Verification items for the finished model (mm, model axes). A direction names the side the tool comes from. Give positions to 0.01 mm unless a question says otherwise; leave off trailing zeros. Write each loop counter-clockwise with the first axis right and the second up, starting at its lowest first coordinate (ties: lowest second). Pieces come first, ordered by that corner, then holes. Notation, with made-up numbers: (-31.5, 89.5) -> (17.5, 89.5) arc R23 ccw to (17.5, 115.5) -> close; hole circle Ø1 at (-20, 54.25). An arc over 180 degrees is marked (long way). Use CSV: the item, a comma, the result in double quotes. Start each with the question number.
```python
from build123d import *

# Parameters (mm, degrees)
F0_R     = 12.5
F1_DEPTH = 20
F2_DEPTH = 45.3


with BuildPart() as f1:
    # F0 (on Front) → F1 (new body)
    with BuildSketch(Plane.XZ):
        with BuildLine():
            ThreePointArc((2.5, 24.874686), (18.540496, 16.77051), (25, 0))
            ThreePointArc((25, 0), (18.540496, -16.77051), (2.5, -24.874686))
            Line((2.5, -24.874686), (101.5, -14.924812))
            ThreePointArc((101.5, -14.924812), (85, 0), (101.5, 14.924812))
            Line((101.5, 14.924812), (2.5, 24.874686))
        make_face()
        with BuildLine():
            ThreePointArc((2.5, -24.874686), (18.540496, -16.77051), (25, 0))
            ThreePointArc((25, 0), (18.540496, 16.77051), (2.5, 24.874686))
            ThreePointArc((2.5, 24.874686), (-25, 0), (2.5, -24.874686))
        make_face()
        with BuildLine():
            ThreePointArc((-11.456439, 5), (0, 12.5), (11.456439, 5))
            Line((11.456439, 5), (15, 5))
            Line((15, 5), (15, -5))
            Line((15, -5), (11.456439, -5))
            ThreePointArc((11.456439, -5), (0, -12.5), (-11.456439, -5))
            Line((-11.456439, -5), (-15, -5))
            Line((-15, -5), (-15, 5))
            Line((-15, 5), (-11.456439, 5))
        make_face(mode=Mode.SUBTRACT)
        with BuildLine():
            ThreePointArc((115, 0), (111.124298, 10.062306), (101.5, 14.924812))
            ThreePointArc((101.5, 14.924812), (85, 0), (101.5, -14.924812))
            ThreePointArc((101.5, -14.924812), (111.124298, -10.062306), (115, 0))
        make_face()
        with Locations((100, 0)):
            Circle(F0_R, mode=Mode.SUBTRACT)
        with BuildLine():
            ThreePointArc((-11.456439, -5), (-12.5, 0), (-11.456439, 5))
            Line((-11.456439, 5), (-15, 5))
            Line((-15, 5), (-15, -5))
            Line((-15, -5), (-11.456439, -5))
        make_face()
    extrude(amount=F1_DEPTH)

    # F0 (on Front) → F2 (join)
    with BuildSketch(Plane.XZ):
        with BuildLine():
            ThreePointArc((2.5, -24.874686), (18.540496, -16.77051), (25, 0))
            ThreePointArc((25, 0), (18.540496, 16.77051), (2.5, 24.874686))
            ThreePointArc((2.5, 24.874686), (-25, 0), (2.5, -24.874686))
        make_face()
        with BuildLine():
            ThreePointArc((-11.456439, 5), (0, 12.5), (11.456439, 5))
            Line((11.456439, 5), (15, 5))
            Line((15, 5), (15, -5))
            Line((15, -5), (11.456439, -5))
            ThreePointArc((11.456439, -5), (0, -12.5), (-11.456439, -5))
            Line((-11.456439, -5), (-15, -5))
            Line((-15, -5), (-15, 5))
            Line((-15, 5), (-11.456439, 5))
        make_face(mode=Mode.SUBTRACT)
        with BuildLine():
            ThreePointArc((-11.456439, -5), (-12.5, 0), (-11.456439, 5))
            Line((-11.456439, 5), (-15, 5))
            Line((-15, 5), (-15, -5))
            Line((-15, -5), (-11.456439, -5))
        make_face()
    extrude(amount=F2_DEPTH)


solid = f1.part
```
(1) Thickness scan on line 1 (X direction, y = -19.5, z = -6); line 2 (Y direction, x = 29, z = 20); line 3 (Z direction, x = 100, y = -13.75). Record the ranges inside material, lowest first. Write a range as from..to.
(2) Draft check along Z on faces 1 (the face through (51, -10, -20)), 2 (the face through (111.923, -9.86, 3.755)), 3 (the face through (15, -22, 0)), 4 (the face through (-11.5, -45.3, 5.9)). Enter one of: released by +Z, released by -Z, zero draft, split by the parting line, or undercut.
(3) Section check C-C on z = -18.5. Record the cut outline in (x, y), then the cut area to 3 significant figures.
(4) Section check A-A on x = 6. Record the cut outline in (y, z).
(5) Go/stop test with flat-tipped pins: pin 1 (1.8 mm diameter, centred on x = 12.5, y = -29, fed in from -Z); pin 2 (6 mm diameter, centred on y = -14.5, z = 6.5, fed in from +X); pin 3 (22.5 mm diameter, centred on x = 100, z = 0, fed in from +Y); pin 4 (25 mm diameter, centred on x = 80.5, z = 9.5, fed in from -Y). Record where each tip stops, or that it passes through.
(6) Section check B-B on y = -15.5. Record the cut outline in (x, z).
(7) Set-up check for faces 5 (the face through (13, -22, 5)), 6 (the face through (28, 0, 0)): record each of +Z, -Z, +X, -X, +Y, -Y from which the full face is reachable in a straight line by a thin tool's end or side.
(8) Section check D-D on x = 20.5. Record the cut outline in (y, z), then the cut area to 3 significant figures.
Data:
1,line 1,"x = -24.27..-10.97, 10.97..89.03, 110.97..113.75"
1,line 2,"y = -20..0"
1,line 3,"z = -15.08..-12.5, 12.5..15.08"
2,face 1,"released by -Z"
2,face 2,"undercut"
2,face 3,"undercut"
2,face 4,"zero draft"
3,outline,"(-16.82, -45.3) -> (16.82, -45.3) -> (16.82, -20) -> (65.93, -20) -> (65.93, 0) -> (-16.82, 0) -> close"
3,area,"2,510 mm2"
4,outline,"(-45.3, -24.27) -> (-20, -24.27) -> (-20, -24.52) -> (0, -24.52) -> (0, -10.97) -> (-45.3, -10.97) -> close; (-45.3, 10.97) -> (0, 10.97) -> (0, 24.52) -> (-20, 24.52) -> (-20, 24.27) -> (-45.3, 24.27) -> close"
5,pin 1,"stops at z = -22.15"
5,pin 2,"stops at x = 114.59"
5,pin 3,"passes through"
5,pin 4,"stops at y = -20"
6,outline,"(2.5, -24.87) -> (101.5, -14.92) arc R15 ccw to (101.5, 14.92) -> (2.5, 24.87) arc R25 ccw (long way) to start; hole (-11.46, -5) arc R12.5 ccw to (11.46, -5) -> (15, -5) -> (15, 5) -> (11.46, 5) arc R12.5 ccw to (-11.46, 5) arc R12.5 ccw to start; hole circle Ø25 at (100, 0)"
7,face 5,"+Y, -Y"
7,face 6,"+Z, -Z, +X, -X, +Y"
8,outline,"(-45.3, -14.31) -> (-20, -14.31) -> (-20, -23.07) -> (0, -23.07) -> (0, 23.07) -> (-20, 23.07) -> (-20, 14.31) -> (-45.3, 14.31) -> close"
8,area,"1,650 mm2"
